For this review, use the dimensioned drawing (mm, ordinates from the lowest corner) and the shaded views. A direction names the side the tool comes from. Coordinates: 2 decimals unless noted, no trailing zeros. Loops run counter-clockwise (first coordinate to the right, second up) from the corner with the lowest first, then second, coordinate; pieces in that order, holes last. Notation, with made-up numbers: M 42,24 L 47,24 A33 ccw 47,63 Z; hole C 56.25,30 d4. An arc over 180 degrees is marked long. Use CSV: the item, a comma, the result in double quotes. Start each with the question number.
1. Tool access review of the marked faces 1, 2, 3 and 4: name each direction out of +Z, -Z, +X, -X, +Y, -Y from which nothing blocks a thin tool from reaching the whole face with its end or side.
2. Add section C-C, the plane y = 17. Write out the cut boundary in (x, z).
3. For L1, parallel to Y at x = 96, z = 22; L2, parallel to Z at x = 77, y = 11; L3, parallel to Z at x = 11, y = 10, list the stretches that pass through material, from the lowest coordinate up.
4. Clearance check with flat-ended pins moving along their axes: P1, Ø4, axis at x = 61.5, y = 63, coming from the +Z side; P2, Ø3, axis at x = 70.5, y = 80.5, coming from the -Z side. State where each tip first meets the part, or that it passes through.
5. Add section A-A, the plane z = 27.5. Write out the cut boundary in (x, y).
6. Draft analysis for pull direction Y (two halves, no side actions). For the marked faces 5, 6 and 7, state which applies: +Y half, -Y half, draft (parallel to the pull), parting line (faces both ways), or undercut.
7. Add section B-B, the plane x = 84. Write out the cut boundary in (y, z).
8. Add section D-D, the plane z = 68. Write out the cut boundary in (x, y).
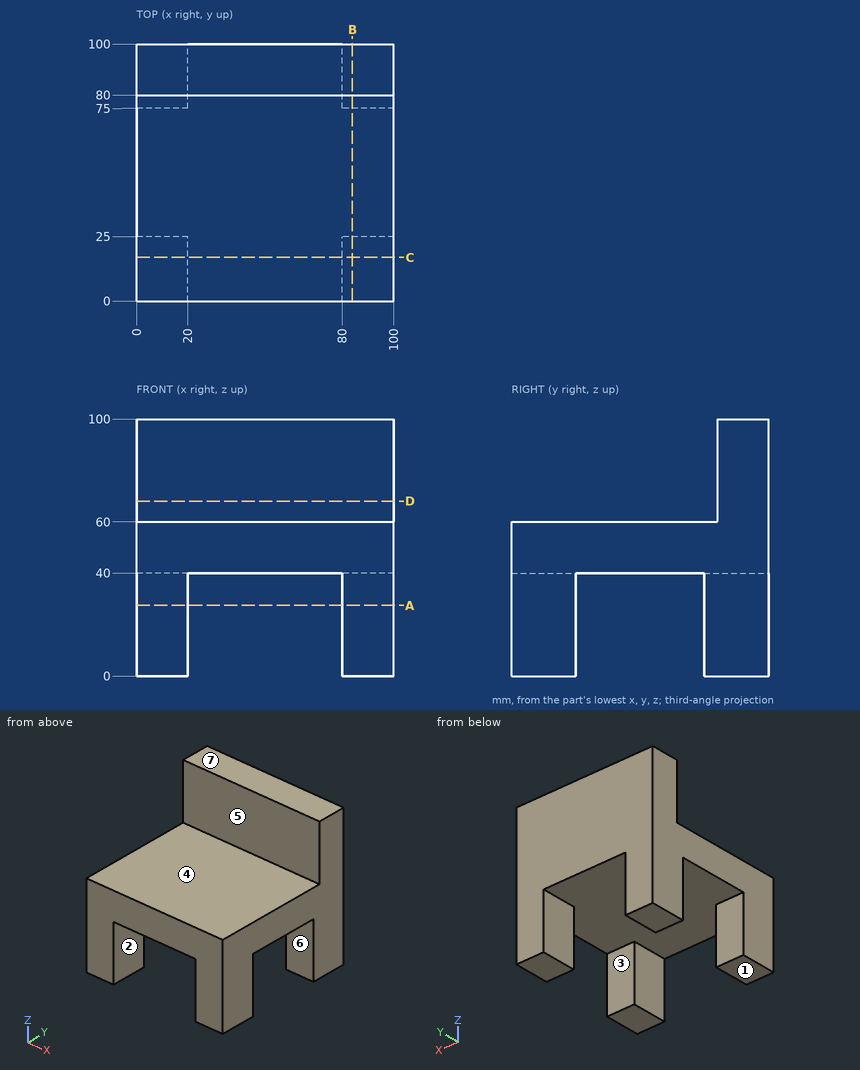
Computed:
1,face 1,"-Z, +X, -X, +Y, -Y"
1,face 2,"-Z, +Y, -Y"
1,face 3,"-Z, +X, -X"
1,face 4,"+Z, +X, -X, -Y"
2,outline,"M 0,0 L 20,0 L 20,40 L 80,40 L 80,0 L 100,0 L 100,60 L 0,60 Z"
3,L1,"y = 0 to 25, 75 to 100"
3,L2,"z = 40 to 60"
3,L3,"z = 0 to 60"
4,P1,"stops at z = 60"
4,P2,"stops at z = 40"
5,outline,"M 0,0 L 20,0 L 20,25 L 0,25 Z; M 0,75 L 20,75 L 20,100 L 0,100 Z; M 80,0 L 100,0 L 100,25 L 80,25 Z; M 80,75 L 100,75 L 100,100 L 80,100 Z"
6,face 5,"-Y half"
6,face 6,"undercut"
6,face 7,"draft"
7,outline,"M 0,0 L 25,0 L 25,40 L 75,40 L 75,0 L 100,0 L 100,100 L 80,100 L 80,60 L 0,60 Z"
8,outline,"M 0,80 L 100,80 L 100,100 L 0,100 Z"
